Source: CAD feature listing. Evaluate the final solid. Frame: model axes, mm. Face numbers are marked on the shaded views. A direction names the side the tool comes from. Give positions to 0.01 mm unless a question says otherwise; leave off trailing zeros. Loops run counter-clockwise (first coordinate to the right, second up) from the corner with the lowest first, then second, coordinate; pieces in that order, holes last. Notation, with made-up numbers: M -29,54 L 18,54 A16 ccw 18,73 Z; hole C 7.5,61 d2. An arc over 180 degrees is marked long. Put each result on its own line as item: value. Start each with the question number.
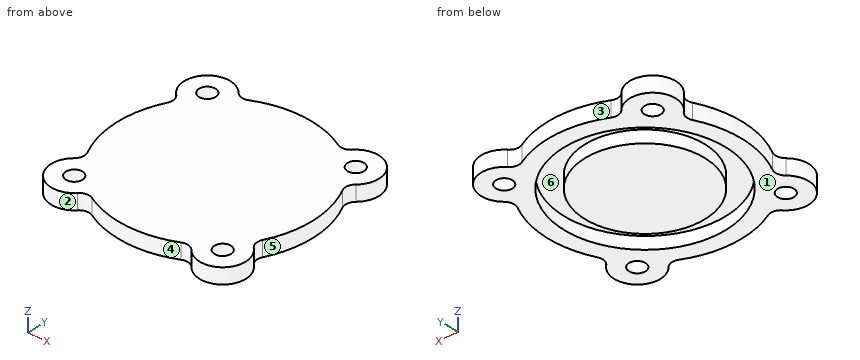
```python
from build123d import *

# Parameters (mm, degrees)
SKETCH_1_R          = 19
EXTRUDE_1_DEPTH     = 3
SKETCH_2_R          = 15.8
SKETCH_2_R_2        = 11.7
CUT_EXTRUDE_1_DEPTH = 2.4
SKETCH_3_R          = 4.5
EXTRUDE_2_DEPTH     = 3
HOLE_WIZARD_M3_1_D  = 3.2
FILLET_1_R          = 2


with BuildPart() as part:
    # ｽｹｯﾁ1 → ﾎﾞｽ - 押し出し1 (new body)
    with BuildSketch(Plane.XY):
        Circle(SKETCH_1_R)
    extrude(amount=EXTRUDE_1_DEPTH)

    # ｽｹｯﾁ2 → ｶｯﾄ - 押し出し1 (cut)
    with BuildSketch(Plane(origin=(0, 0, 0), x_dir=(-1, 0, 0), z_dir=(0, 0, -1))):
        Circle(SKETCH_2_R)
        Circle(SKETCH_2_R_2, mode=Mode.SUBTRACT)
    extrude(amount=-CUT_EXTRUDE_1_DEPTH, mode=Mode.SUBTRACT)

    # ｽｹｯﾁ3 → ﾎﾞｽ - 押し出し2 (add)
    with BuildSketch(Plane.XY.offset(3)):
        with Locations((-14.354267658, 14.354267658)):
            Circle(SKETCH_3_R)
        with Locations((14.354267658, 14.354267658)):
            Circle(SKETCH_3_R)
        with Locations((14.354267658, -14.354267658)):
            Circle(SKETCH_3_R)
        with Locations((-14.354267658, -14.354267658)):
            Circle(SKETCH_3_R)
    extrude(amount=-EXTRUDE_2_DEPTH)

    # M3 すきま穴1 (through all)
    with Locations(Plane.XY.offset(3)):
        with Locations((-14.354267658, 14.354267658), (-14.354267658, -14.354267658), (14.354267658, 14.354267658), (14.354267658, -14.354267658)):
            Hole(HOLE_WIZARD_M3_1_D / 2)

    # ﾌｨﾚｯﾄ1
    fillet_1_edges = [part.edges().sort_by_distance(p)[0] for p in [
        (-10.182407316, 16.041152741, 1.5),
        (-16.041152741, 10.182407316, 1.5),
        (16.041152741, 10.182407316, 1.5),
        (10.182407316, 16.041152741, 1.5),
        (10.182407316, -16.041152741, 1.5),
        (16.041152741, -10.182407316, 1.5),
        (-16.041152741, -10.182407316, 1.5),
        (-10.182407316, -16.041152741, 1.5),
    ]]
    fillet(fillet_1_edges, radius=FILLET_1_R)


solid = part.part
```
1. Ray query, line 1 (X direction, y = 7, z = 0.65); line 2 (Y direction, x = 4, z = 0.3) (3 decimals); line 3 (Y direction, x = 10.5, z = 1.4). Return the intervals inside material, ascending.
2. Section C-C, the plane x = 5.5. Output: boundary loops of the cut face in (y, z).
3. Contact query for flat-ended pins moving along their axis: pin 1 (6 mm diameter, centred on x = 9.5, y = -14, fed in from -Z); pin 2 (1 mm diameter, centred on x = 9, z = 1.5, fed in from -Y). Output: stop coordinate, or through.
4. Section A-A, the plane x = 14.5. Output: boundary loops of the cut face in (y, z).
5. Pull-direction query (Y, two-part tool) for the marked faces 1, 2, 3 and 4; classes: released by +Y, released by -Y, zero draft, split by the parting line, or undercut.
6. Set-up query: the marked faces 5 and 6. Return all of +Z, -Z, +X, -X, +Y, -Y with unobstructed straight access to the full face (end or side cutting, diameter ignored); none if empty.
7. Section B-B, the plane y = 0. Output: boundary loops of the cut face in (x, z).
8. Section D-D, the plane z = 1.6. State how many separate pieces and enclosed holes the cut face has, plus the area to 3 significant figures.
Results found:
1. line 1: -17.66 to -14.16, -9.37 to 9.37, 14.16 to 17.66
1. line 2: -18.574 to -15.285, -10.995 to 10.995, 15.285 to 18.574
1. line 3: -16.96 to -11.81, -5.16 to 5.16, 11.81 to 16.96
2. outline: M -18.19,0 L -14.81,0 L -14.81,2.4 L -10.33,2.4 L -10.33,0 L 10.33,0 L 10.33,2.4 L 14.81,2.4 L 14.81,0 L 18.19,0 L 18.19,3 L -18.19,3 Z
3. pin 1: z = 0
3. pin 2: y = -16.99
4. outline: M -18.85,0 L -15.95,0 L -15.95,3 L -18.85,3 Z; M -12.76,0 L -6.28,0 L -6.28,2.4 L 6.28,2.4 L 6.28,0 L 12.76,0 L 12.76,3 L -12.76,3 Z; M 15.95,0 L 18.85,0 L 18.85,3 L 15.95,3 Z
5. face 1: zero draft
5. face 2: undercut
5. face 3: released by +Y
5. face 4: released by -Y
6. face 5: +Z, -Z, +X
6. face 6: -Z
7. outline: M -19,0 L -15.8,0 L -15.8,2.4 L -11.7,2.4 L -11.7,0 L 11.7,0 L 11.7,2.4 L 15.8,2.4 L 15.8,0 L 19,0 L 19,3 L -19,3 Z
8. separate pieces: 2
8. enclosed holes: 5
8. area: 931 mm²
